Input: dimensioned drawing with shaded views. Units: mm. Origin: part minimum x, y, z. A direction names the side the tool comes from. Coordinates: 2 decimals unless noted, no trailing zeros. Order: outer loops, then holes, each group sorted by start corner. A loop starts at its lowest first (then second) coordinate and runs counter-clockwise, first axis right, second up. Notation, with made-up numbers: M 16.5,74.25 L 58.5,74.25 A14 cw 58.5,91.25 Z; hole C 16,16.5 d2. An arc over 180 degrees is marked long. Use CSV: the item, a comma, the result in double quotes. Start each with the question number.
1. Section query A-A on z = 25. Return the cut outline in (x, y).
2. Section query D-D on z = 42.5. Return the cut outline in (x, y).
3. Material intervals for line 1 (X direction, y = 6, z = 25); line 2 (X direction, y = 21.5, z = 28.5); line 3 (X direction, y = 14.5, z = 23), sorted ascending.
4. Section query C-C on y = 24. Return the cut outline in (x, z).
5. First-contact query: P1, Ø16, axis at x = 82.5, z = 25, coming from the +Y side; P2, Ø9, axis at x = 12.5, z = 25, coming from the -Y side. Flat tips, straight axial feed; report the tip coordinate or a pass-through.
6. Section query B-B on x = 8.5. Return the cut outline in (y, z), and give its area (3 significant figures).
7. Set-up query: the marked faces 1, 2 and 3. Return all of +Z, -Z, +X, -X, +Y, -Y with unobstructed straight access to the full face (end or side cutting, diameter ignored); none if empty.
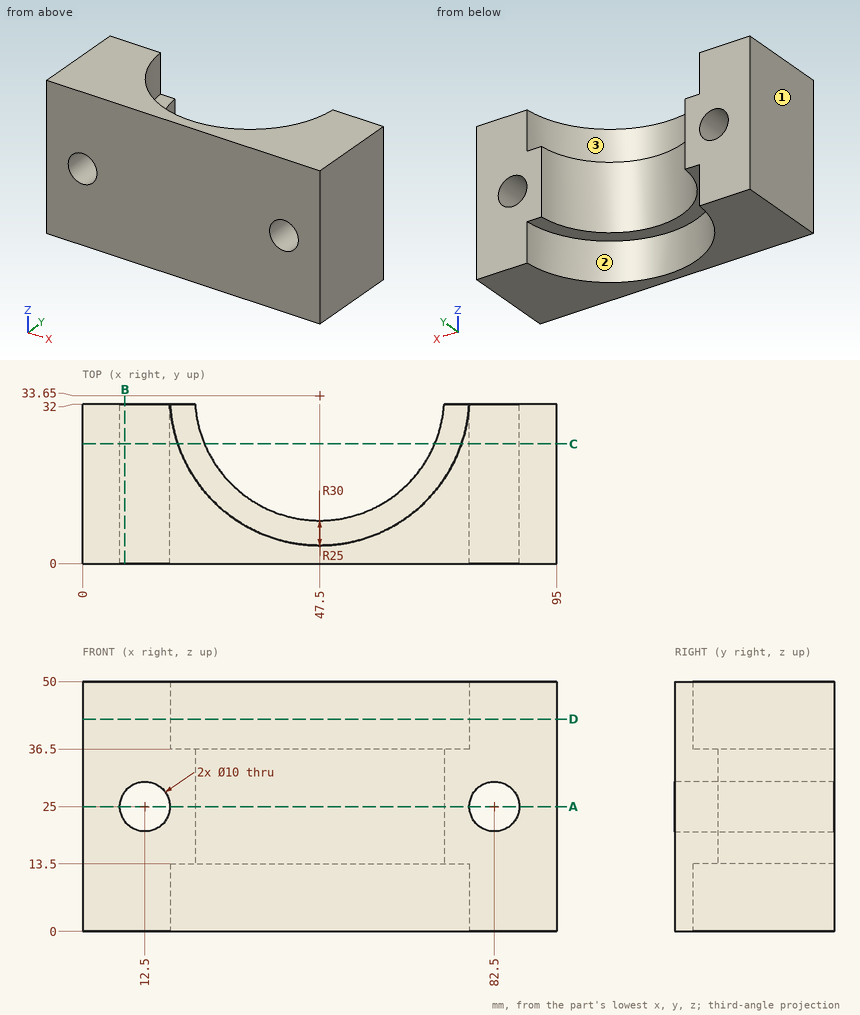
Results list:
1,outline,"M 0,0 L 7.5,0 L 7.5,32 L 0,32 Z; M 17.5,0 L 77.5,0 L 77.5,32 L 72.45,32 A25 cw 22.55,32 L 17.5,32 Z; M 87.5,0 L 95,0 L 95,32 L 87.5,32 Z"
2,outline,"M 0,0 L 95,0 L 95,32 L 77.45,32 A30 cw 17.55,32 L 0,32 Z"
3,line 1,"x = 0 to 7.5, 17.5 to 77.5, 87.5 to 95"
3,line 2,"x = 0 to 8.93, 16.07 to 25.65, 69.35 to 78.93, 86.07 to 95"
3,line 3,"x = 0 to 7.92, 17.08 to 31.43, 63.57 to 77.92, 87.08 to 95"
4,outline,"M 0,0 L 19.09,0 L 19.09,13.5 L 24.44,13.5 L 24.44,36.5 L 19.09,36.5 L 19.09,50 L 0,50 Z; M 70.56,13.5 L 75.91,13.5 L 75.91,0 L 95,0 L 95,50 L 75.91,50 L 75.91,36.5 L 70.56,36.5 Z; hole C 12.5,25 d10; hole C 82.5,25 d10"
5,P1,"stops at y = 32"
5,P2,"passes through"
6,outline,"M 0,0 L 32,0 L 32,22 L 0,22 Z; M 0,28 L 32,28 L 32,50 L 0,50 Z"
6,area,"1,410 mm²"
7,face 1,"+Z, -Z, -X, +Y, -Y"
7,face 2,"-Z, +Y"
7,face 3,"+Z, +Y"
